For this review, take the finished solid that the model builds, in its own axes (mm). Face numbers are marked on the shaded views. A direction names the side the tool comes from. Give positions to 0.01 mm unless a question says otherwise; leave off trailing zeros. Write each loop counter-clockwise with the first axis right and the second up, starting at its lowest first coordinate (ties: lowest second). Pieces come first, ordered by that corner, then holes.
Q1. We need section C-C (x = 4.5). Write out the cut boundary in (y, z).
Q2. For line 1 (X direction, y = -29.5, z = -41); line 2 (Z direction, x = 62, y = -23); line 3 (X direction, y = -37.5, z = -102), list the stretches that pass through material, from the lowest coordinate up.
Q3. Machinability: for the marked faces 4 and 5, which of the approach directions +Z, -Z, +X, -X, +Y, -Y give a long, thin tool a straight path to every point of the face, cutting with its end or side? Answer none if there is none.
Q4. We need section B-B (x = 38.38). Write out the cut boundary in (y, z), then the cut area to 3 significant figures.
Q5. We need section D-D (z = 95). Write out the cut boundary in (x, y), then the cut area to 3 significant figures.
Q6. Mouldability with a two-part tool opening along X and no side actions: class the marked faces 1, 2 and 3 as released by +X, released by -X, zero draft, split by the parting line, or undercut.
Q7. We need section A-A (z = 12.5). Write out the cut boundary in (x, y), then the cut area to 3 significant figures.
Q8. Insertion check: P1, Ø8, axis at x = 9.5, z = -8, coming from the +Y side; P2, Ø5, axis at x = -62.5, z = 112.5, coming from the -Y side. Each pin has a flat end and moves straight along its axis. Give the tip position at first contact, or say it passes through.
```python
from build123d import *

# Parameters (mm, degrees)
SKETCH1_W              = 150
SKETCH1_H              = 250
BOSS_EXTRUDE1_DEPTH    = 40
CUT_EXTRUDE1_REACH     = 153.162
SKETCH3_W              = 58
SKETCH3_H              = 85
SKETCH3_W_2            = 47
FILLET1_R              = 10
SKETCH7_R              = 7.5
CUT_EXTRUDE4_DEPTH     = 369.774778015
SKETCH8_R              = 10
CUT_EXTRUDE5_DEPTH     = 30
M10_TAPPED_HOLE1_D     = 8.5
M10_TAPPED_HOLE1_DEPTH = 24.5
M10_TAPPED_HOLE1_TIP   = 2.553657631
F_10_0MM_DOWEL_HOLE1_D = 10
CUT_EXTRUDE6_REACH     = 153.162
SKETCH15_R             = 7.5
SKETCH16_R             = 9
CUT_EXTRUDE7_DEPTH     = 30


with BuildPart() as part:
    # Sketch1 → Boss-Extrude1 (new body)
    with BuildSketch(Plane(origin=(0, 0, 0), x_dir=(1, 0, 0), z_dir=(0, 1, 0))):
        Rectangle(SKETCH1_W, SKETCH1_H)
    extrude(amount=-BOSS_EXTRUDE1_DEPTH)

    # Sketch3 → Cut-Extrude1 (cut, up to next)
    with BuildSketch(Plane(origin=(0, 0, 0), x_dir=(1, 0, 0), z_dir=(0, 1, 0)), mode=Mode.PRIVATE) as cut_extrude1_sk1:
        with Locations((-27.25, 7.73)):
            Rectangle(SKETCH3_W, SKETCH3_H)
    cut_extrude1_tool1 = extrude(cut_extrude1_sk1.sketch, amount=-CUT_EXTRUDE1_REACH, mode=Mode.PRIVATE) & part.part
    # Sketch3 → Cut-Extrude1 (cut, up to next)
    with BuildSketch(Plane(origin=(0, 0, 0), x_dir=(1, 0, 0), z_dir=(0, 1, 0)), mode=Mode.PRIVATE) as cut_extrude1_sk2:
        with Locations((33.25, 7.73)):
            Rectangle(SKETCH3_W_2, SKETCH3_H)
    cut_extrude1_tool2 = extrude(cut_extrude1_sk2.sketch, amount=-CUT_EXTRUDE1_REACH, mode=Mode.PRIVATE) & part.part
    add(cut_extrude1_tool1.solids().sort_by_distance((-27.25, 0, -7.73))[0], mode=Mode.SUBTRACT)
    add(cut_extrude1_tool2.solids().sort_by_distance((33.25, 0, -7.73))[0], mode=Mode.SUBTRACT)

    # Fillet1
    fillet1_edges = [part.edges().sort_by_distance(p)[0] for p in [
        (-56.25, -20, 34.77),
        (-56.25, -20, -50.23),
        (1.75, -20, -50.23),
        (1.75, -20, 34.77),
        (9.75, -20, 34.77),
        (9.75, -20, -50.23),
        (56.75, -20, -50.23),
        (56.75, -20, 34.77),
    ]]
    fillet(fillet1_edges, radius=FILLET1_R)

    # Sketch7 → Cut-Extrude4 (cut, through all)
    with BuildSketch(Plane(origin=(269.63, 0, 0), x_dir=(1, 0, 0), z_dir=(0, 1, 0))):
        with Locations((-263.88, 10.23)):
            Circle(SKETCH7_R)
    extrude(amount=-CUT_EXTRUDE4_DEPTH, mode=Mode.SUBTRACT)

    # Sketch8 → Cut-Extrude5 (cut)
    with BuildSketch(Plane(origin=(269.63, -40, 0), x_dir=(1, 0, 0), z_dir=(0, -1, 0))):
        with Locations((-263.88, -10.23)):
            Circle(SKETCH8_R)
    extrude(amount=-CUT_EXTRUDE5_DEPTH, mode=Mode.SUBTRACT)

    # M10 Tapped Hole1
    with Locations(Plane(origin=(0, -40, 0), x_dir=(-1, 0, 0), z_dir=(0, -1, 0))):
        with Locations((-62.5, 112.5), (62.5, 112.5), (62.5, -112.5), (-62.5, -112.5)):
            Hole(M10_TAPPED_HOLE1_D / 2, depth=M10_TAPPED_HOLE1_DEPTH)
            with Locations((0, 0, -(M10_TAPPED_HOLE1_DEPTH + M10_TAPPED_HOLE1_TIP / 2))):  # 118° drill point
                Cone(0, M10_TAPPED_HOLE1_D / 2, M10_TAPPED_HOLE1_TIP, mode=Mode.SUBTRACT)

    # Ø10.0mm Dowel Hole1 (through all)
    with Locations(Plane(origin=(0, -40, 0), x_dir=(-1, 0, 0), z_dir=(0, -1, 0))):
        with Locations((-62.5, 95), (-62.5, -95), (62.5, -95), (62.5, 95)):
            Hole(F_10_0MM_DOWEL_HOLE1_D / 2)

    # Sketch15 → Cut-Extrude6 (cut, up to next)
    with BuildSketch(Plane(origin=(0, 0, 0), x_dir=(1, 0, 0), z_dir=(0, 1, 0)), mode=Mode.PRIVATE) as cut_extrude6_sk1:
        with Locations(Location((38.38, -99.376818869, 0), (0, 0, 270))):
            Circle(SKETCH15_R)
    cut_extrude6_tool1 = extrude(cut_extrude6_sk1.sketch, amount=-CUT_EXTRUDE6_REACH, mode=Mode.PRIVATE) & part.part
    # Sketch15 → Cut-Extrude6 (cut, up to next)
    with BuildSketch(Plane(origin=(0, 0, 0), x_dir=(1, 0, 0), z_dir=(0, 1, 0)), mode=Mode.PRIVATE) as cut_extrude6_sk2:
        with Locations(Location((-37.87, -99.370796223, 0), (0, 0, 270))):
            Circle(SKETCH15_R)
    cut_extrude6_tool2 = extrude(cut_extrude6_sk2.sketch, amount=-CUT_EXTRUDE6_REACH, mode=Mode.PRIVATE) & part.part
    # Sketch15 → Cut-Extrude6 (cut, up to next)
    with BuildSketch(Plane(origin=(0, 0, 0), x_dir=(1, 0, 0), z_dir=(0, 1, 0)), mode=Mode.PRIVATE) as cut_extrude6_sk3:
        with Locations(Location((38.38, 99.376818869, 0), (0, 0, 270))):
            Circle(SKETCH15_R)
    cut_extrude6_tool3 = extrude(cut_extrude6_sk3.sketch, amount=-CUT_EXTRUDE6_REACH, mode=Mode.PRIVATE) & part.part
    # Sketch15 → Cut-Extrude6 (cut, up to next)
    with BuildSketch(Plane(origin=(0, 0, 0), x_dir=(1, 0, 0), z_dir=(0, 1, 0)), mode=Mode.PRIVATE) as cut_extrude6_sk4:
        with Locations(Location((-37.87, 99.370796223, 0), (0, 0, 270))):
            Circle(SKETCH15_R)
    cut_extrude6_tool4 = extrude(cut_extrude6_sk4.sketch, amount=-CUT_EXTRUDE6_REACH, mode=Mode.PRIVATE) & part.part
    add(cut_extrude6_tool1.solids().sort_by_distance((38.38, 0, 99.376819))[0], mode=Mode.SUBTRACT)
    add(cut_extrude6_tool2.solids().sort_by_distance((-37.87, 0, 99.370796))[0], mode=Mode.SUBTRACT)
    add(cut_extrude6_tool3.solids().sort_by_distance((38.38, 0, -99.376819))[0], mode=Mode.SUBTRACT)
    add(cut_extrude6_tool4.solids().sort_by_distance((-37.87, 0, -99.370796))[0], mode=Mode.SUBTRACT)

    # Sketch16 → Cut-Extrude7 (cut)
    with BuildSketch(Plane.XZ.offset(40)):
        with Locations(Location((-37.87, -99.370796223, 0), (0, 0, 270))):
            Circle(SKETCH16_R)
        with Locations(Location((38.38, -99.376818869, 0), (0, 0, 270))):
            Circle(SKETCH16_R)
        with Locations(Location((38.38, 99.376818869, 0), (0, 0, 270))):
            Circle(SKETCH16_R)
        with Locations(Location((-37.87, 99.370796223, 0), (0, 0, 270))):
            Circle(SKETCH16_R)
    extrude(amount=-CUT_EXTRUDE7_DEPTH, mode=Mode.SUBTRACT)


solid = part.part
```
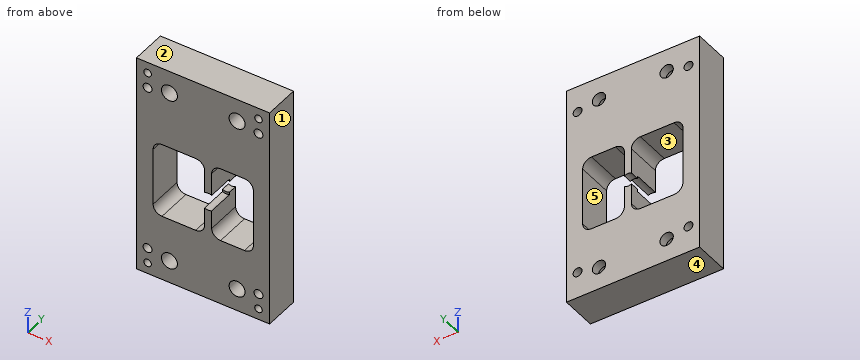
Computed:
1. outline: (-40, -125) - (0, -125) - (0, -17.63) - (-10, -17.63) - (-10, -20.15) - (-40, -20.15) - close; (-40, -0.31) - (-10, -0.31) - (-10, -2.83) - (0, -2.83) - (0, 125) - (-40, 125) - close
2. line 1: x = -75 to -56.22, 1.72 to 9.78, 56.72 to 75
2. line 2: z = -125 to -116.72, -108.28 to -99.97, -90.03 to 90.03, 99.97 to 108.28, 116.72 to 125
2. line 3: x = -75 to -46.48, -29.26 to 29.77, 46.99 to 75
3. face 4: -Z, +X, -X, +Y, -Y
3. face 5: +Y, -Y
4. outline: (-40, -125) - (0, -125) - (0, -106.88) - (-10, -106.88) - (-10, -108.38) - (-40, -108.38) - close; (-40, -90.38) - (-10, -90.38) - (-10, -91.88) - (0, -91.88) - (0, -50.23) - (-40, -50.23) - close; (-40, 34.77) - (0, 34.77) - (0, 91.88) - (-10, 91.88) - (-10, 90.38) - (-40, 90.38) - close; (-40, 108.38) - (-10, 108.38) - (-10, 106.88) - (0, 106.88) - (0, 125) - (-40, 125) - close
4. area: 5,220 mm2
5. outline: (-75, -40) - (-67.5, -40) - (-67.5, 0) - (-75, 0) - close; (-57.5, -40) - (-45.74, -40) - (-45.74, -10) - (-43.96, -10) - (-43.96, 0) - (-57.5, 0) - close; (-31.78, -10) - (-30, -10) - (-30, -40) - (30.52, -40) - (30.52, -10) - (32.29, -10) - (32.29, 0) - (-31.78, 0) - close; (44.47, -10) - (46.24, -10) - (46.24, -40) - (57.5, -40) - (57.5, 0) - (44.47, 0) - close; (67.5, -40) - (75, -40) - (75, 0) - (67.5, 0) - close
5. area: 4,010 mm2
6. face 1: released by +X
6. face 2: zero draft
6. face 3: undercut
7. outline: (-75, -40) - (-56.25, -40) - (-56.25, 0) - (-75, 0) - close; (1.75, -40) - (9.75, -40) - (9.75, 0) - (1.75, 0) - close; (56.75, -40) - (75, -40) - (75, 0) - (56.75, 0) - close
7. area: 1,800 mm2
8. P1: passes through
8. P2: stops at y = -14.45
